The model under review builds one solid part; all positions refer to its coordinate system, in mm. A direction names the side the tool comes from. Round coordinates to 2 decimals unless told otherwise and drop trailing zeros. Order: outer loops, then holes, each group sorted by start corner. A loop starts at its lowest first (then second) coordinate and runs counter-clockwise, first axis right, second up.
1) To check wall thickness, follow L1, parallel to Y at x = 50.8, z = 5.5; L2, parallel to X at y = -5.25, z = 41.5. State the ranges of each line that lie inside material, in increasing order.
2) Mouldability with a two-part tool opening along Y and no side actions: class faces 1 (the face through (6, -19.033, 43)), 2 (the face through (6, -6.35, 44)), 3 (the face through (6.44, -1.75, 44.53)), 4 (the face through (22, -25.4, 11)) as pulls with the +Y half, pulls with the -Y half, needs draft (parallel to the pull), parting line crosses it, or undercut.
3) Consider section B-B (z = 36). Give the boundary of the cut face in (x, y).
4) Consider section D-D (x = 10.5). Give the boundary of the cut face in (y, z), then the cut area to 3 significant figures.
5) Consider section C-C (y = -16.75). Give the boundary of the cut face in (x, z).
6) Consider section A-A (x = 50.8). Give the boundary of the cut face in (y, z).
7) Machinability: for faces 5 (the face through (42, -13, 12.7)), 6 (the face through (6.44, -23.74, 44.38)), which of the approach directions +Z, -Z, +X, -X, +Y, -Y give a long, thin tool a straight path to every point of the face, cutting with its end or side? Answer none if there is none.
8) Clearance check with flat-ended pins moving along their axes: P1, Ø10, axis at x = 25.4, y = -12.7, coming from the +Z side; P2, Ø5.5, axis at x = 7, z = 44, coming from the +Y side; P3, Ø3, axis at x = 36, y = -19.5, coming from the +Z side; P4, Ø3.5, axis at x = 6.5, z = 42, coming from the -Y side. State where each tip first meets the part, or that it passes through.
from build123d import *

# Parameters (mm, degrees)
F1_DEPTH = 25.4
F2_R     = 6.35
F3_DEPTH = 25.4
F5_DEPTH = 25.4
F7_DEPTH = 25.4


with BuildPart() as f1:
    # F0 (on Front) → F1 (new body)
    with BuildSketch(Plane.XZ):
        Polygon((12.7, 50.8), (0, 50.8), (0, 0), (69.85, 0), (69.85, 12.7), (12.7, 12.7), align=None)
    extrude(amount=F1_DEPTH)

    # F2 (on face) → F3 (cut)
    with BuildSketch(Plane.XY.offset(12.7)):
        with Locations((25.4, -12.7)):
            Circle(F2_R)
        with BuildLine():
            Line((69.85, -25.4), (69.85, -12.7))
            ThreePointArc((69.85, -12.7), (66.1302561211, -21.6802561211), (57.15, -25.4))
            Line((57.15, -25.4), (69.85, -25.4))
        make_face()
        with Locations((50.8, -12.7)):
            Circle(F2_R)
        with BuildLine():
            Line((69.85, 0), (57.15, 0))
            ThreePointArc((57.15, 0), (66.1302561211, -3.7197438789), (69.85, -12.7))
            Line((69.85, -12.7), (69.85, 0))
        make_face()
    extrude(amount=-F3_DEPTH, mode=Mode.SUBTRACT)

    # F4 (on face) → F5 (cut)
    with BuildSketch(Plane.YZ.offset(12.7)):
        with BuildLine():
            Line((0, 38.1), (0, 39.259262383))
            Line((0, 39.259262383), (0, 50.8))
            Line((0, 50.8), (-12.7, 50.8))
            ThreePointArc((-12.7, 50.8), (-3.7197438789, 47.0802561211), (0, 38.1))
        make_face()
        with BuildLine():
            ThreePointArc((-25.4, 38.1), (-21.6802561211, 47.0802561211), (-12.7, 50.8))
            Line((-12.7, 50.8), (-25.4, 50.8))
            Line((-25.4, 50.8), (-25.4, 39.259262383))
            Line((-25.4, 39.259262383), (-25.4, 38.1))
        make_face()
    extrude(amount=-F5_DEPTH, mode=Mode.SUBTRACT)

    # F6 (on face) → F7 (cut)
    with BuildSketch(Plane.YZ.offset(12.7)):
        with BuildLine():
            Line((-19.0331310429, 38.5625485848), (-19.0331310429, 37.6374514152))
            ThreePointArc((-19.0331310429, 37.6374514152), (-12.4685719577, 31.7542186406), (-6.35, 38.1))
            ThreePointArc((-6.35, 38.1), (-12.4685719577, 44.4457813594), (-19.0331310429, 38.5625485848))
        make_face()
        with BuildLine():
            ThreePointArc((-19.0331310429, 38.5625485848), (-12.4685719577, 44.4457813594), (-6.35, 38.1))
            Line((-6.35, 38.1), (-6.35, 49.0985226281))
            ThreePointArc((-6.35, 49.0985226281), (-12.6902650085, 50.7999962689), (-19.0331310429, 49.1082446917))
            Line((-19.0331310429, 49.1082446917), (-19.0331310429, 38.5625485848))
        make_face()
    extrude(amount=-F7_DEPTH, mode=Mode.SUBTRACT)


solid = f1.part
Answer below:
1. L1: y = -25.4 to -19.05, -6.35 to 0
1. L2: x = 0 to 12.7
2. face 1: undercut
2. face 2: undercut
2. face 3: pulls with the +Y half
2. face 4: pulls with the -Y half
3. outline: (0, -25.4) - (12.7, -25.4) - (12.7, -18.69) - (0, -18.69) - close; (0, -6.71) - (12.7, -6.71) - (12.7, 0) - (0, 0) - close
4. outline: (-25.4, 0) - (0, 0) - (0, 38.1) arc R12.7 ccw to (-6.35, 49.1) - (-6.35, 38.1) arc R6.35 cw to (-19.03, 37.64) - (-19.03, 49.11) arc R12.7 ccw to (-25.4, 38.1) - close
4. area: 1,000 mm2
5. outline: (0, 0) - (20.51, 0) - (20.51, 12.7) - (12.7, 12.7) - (12.7, 33.21) - (0, 33.21) - close; (30.29, 0) - (45.91, 0) - (45.91, 12.7) - (30.29, 12.7) - close; (55.69, 0) - (69.19, 0) - (69.19, 12.7) - (55.69, 12.7) - close
6. outline: (-25.4, 0) - (-19.05, 0) - (-19.05, 12.7) - (-25.4, 12.7) - close; (-6.35, 0) - (0, 0) - (0, 12.7) - (-6.35, 12.7) - close
7. face 5: +Z, +X, +Y, -Y
7. face 6: +Z, +X, -X, -Y
8. P1: passes through
8. P2: stops at y = -0.4
8. P3: stops at z = 12.7
8. P4: stops at y = -25.22
